Geometry check sheet. Reference: the model listing, model coordinates, mm. Face numbers are marked on the shaded views. A direction names the side the tool comes from. Coordinates: 2 decimals unless noted, no trailing zeros. Order: outer loops, then holes, each group sorted by start corner. A loop starts at its lowest first (then second) coordinate and runs counter-clockwise, first axis right, second up.
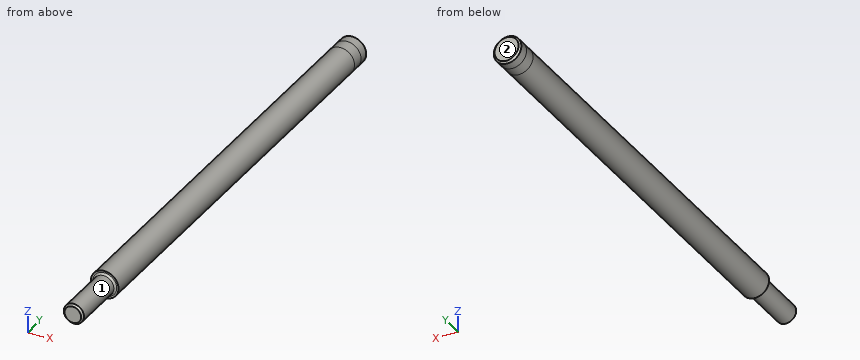
Autodesk Inventor part; units mm, degrees
ref_plane "YZ Plane" through (0, 0, 0) normal (1, 0, 0) x (0, 1, 0)
ref_plane "XZ Plane" through (0, 0, 0) normal (0, 1, 0) x (-1, 0, 0)
ref_plane "XY Plane" through (0, 0, 0) normal (0, 0, 1) x (1, 0, 0)
sketch "Sketch1" plane through (0, 0, 0) normal (0, 1, 0) x (-1, 0, 0)
  circle A0 centre (0, 0) radius 15
  dimension "d0" = 30
extrude "Extrusion1" add sketch "Sketch1" along normal blind 459
sketch "Sketch2" plane through (0, 0, 0) normal (0, -1, 0) x (1, 0, 0)
  circle A0 centre (0, 0) radius 11
  dimension "d3" = 22
extrude "Extrusion2" add sketch "Sketch2" along normal blind 62
fillet "Fillet1" radius 2 1 edges at (-11, 0, 0)
sketch "Sketch3" plane through (0, 459, 0) normal (0, 1, 0) x (1, 0, 0)
  circle A0 centre (0, 0) radius 15
  dimension "d7" = 30
extrude "Extrusion3" add sketch "Sketch3" along normal blind 12.7
thread "Thread2"
sketch "Sketch4" plane through (0, 471.7, 0) normal (0, 1, 0) x (1, 0, 0)
  circle A0 centre (0, 0) radius 15
extrude "Extrusion4" add sketch "Sketch4" along normal blind 12
thread "Thread3"
chamfer "Chamfer1" distance 2 angle 45 1 edges at (-15, 483.7, 0)
chamfer "Chamfer2" distance 2 angle 45 1 edges at (-11, -62, 0)
properties part number "BARRA SOPORTE"
Item 1: Sectioned sample at A-A (x = 0). Record the cut outline in (y, z).
Item 2: Depth check by flat-ended pin: P1, Ø6, axis at y = 175, z = 8.5, coming from the -X side; P2, Ø2, axis at x = -9, y = 255, coming from the +Z side; P3, Ø4, axis at x = -7.5, y = 389, coming from the -Z side. Enter the tip coordinate at first touch or a pass-through.
Item 3: Sectioned sample at C-C (y = 191). Record the cut outline in (x, z), and give its area (3 significant figures).
Item 4: Sectioned sample at B-B (z = 0). Record the cut outline in (x, y), and give its area (3 significant figures).
Item 5: Tool access check on the marked faces 1 and 2. Record the directions out of +Z, -Z, +X, -X, +Y, -Y that give a thin tool (end or side, any length) a straight path to the whole face; none if there is none.
Item 6: Thickness scan on line 1 along Y through (x, z) = (-10.5, 6.75); line 2 along Z through (x, y) = (1, -15); line 3 along X through (y, z) = (158, 1). Record the ranges inside material, lowest first.
Geometry check:
1. outline: (-62, -9) - (-60, -11) - (-2, -11) arc R2 cw to (0, -13) - (0, -15) - (481.7, -15) - (483.7, -13) - (483.7, 13) - (481.7, 15) - (0, 15) - (0, 13) arc R2 cw to (-2, 11) - (-60, 11) - (-62, 9) - close
2. P1: stops at x = -13.96
2. P2: stops at z = 12.69
2. P3: stops at z = -13.96
3. outline: circle Ø30 at (0, 0)
3. area: 707 mm2
4. outline: (-15, 0) - (-13, 0) arc R2 cw to (-11, -2) - (-11, -60) - (-9, -62) - (9, -62) - (11, -60) - (11, -2) arc R2 cw to (13, 0) - (15, 0) - (15, 481.7) - (13, 483.7) - (-13, 483.7) - (-15, 481.7) - close
4. area: 15,900 mm2
5. face 1: -Y
5. face 2: +Z, -Z, +X, -X, +Y
6. line 1: y = -0.07 to 483.7
6. line 2: z = -10.95 to 10.95
6. line 3: x = -14.97 to 14.97
